Answer from the drawing. Dimensions are ordinates in mm from the lowest x, y and z of the part. A direction names the side the tool comes from. Give positions to 0.01 mm unless a question says otherwise; leave off trailing zeros. Write each loop counter-clockwise with the first axis right and the second up, starting at its lowest first coordinate (ties: lowest second). Pieces come first, ordered by that corner, then holes. Notation, with made-up numbers: (87.5, -9.5) -> (126.5, -9.5) arc R30 ccw to (126.5, 15.5) -> close; hole circle Ø2 at (10, 44). An arc over 180 degrees is marked (long way). Put each result on its own line as item: value. Start each with the question number.
1) A cutting plane is placed at A-A (z = 4.6). Write down the section's boundary in (x, y) (1 decimal), then the cut area to 3 significant figures.
2) Flat-ended cylindrical pins translate along their axes: pin 1 Ø1 at (x, z) = (11, 4) entering from -Y; pin 2 Ø3 at (x, y) = (5.5, 6.5) entering from +Z; pin 3 Ø1 at (x, y) = (9, 8.5) entering from +Z. Find the tip coordinate at first contact, or state that the pin passes through.
3) For the marked faces 1 and 2, determine the directions among +Z, -Z, +X, -X, +Y, -Y from which every point of the face is accessible in a straight line to the end or side of a thin tool.
4) A cutting plane is placed at C-C (x = 13.5). Write down the section's boundary in (y, z) (1 decimal), then the cut area to 3 significant figures.
5) A cutting plane is placed at D-D (x = 11.25). Write down the section's boundary in (y, z) (1 decimal).
6) Find the intervals of material crossed by line 1 along Y through (x, z) = (6.5, 4) (1 decimal); line 2 along X through (y, z) = (3.25, 3.3) (1 decimal); line 3 along X through (y, z) = (6.5, 0.7) (1 decimal), in increasing order. Write a range as from..to.
7) For a pull along X with two mould halves and no side action, classify the marked faces 3, 4, 5 and 6 as released by +X, released by -X, zero draft, split by the parting line, or undercut.
8) A cutting plane is placed at B-B (y = 8). Write down the section's boundary in (x, z) (1 decimal), then the cut area to 3 significant figures.
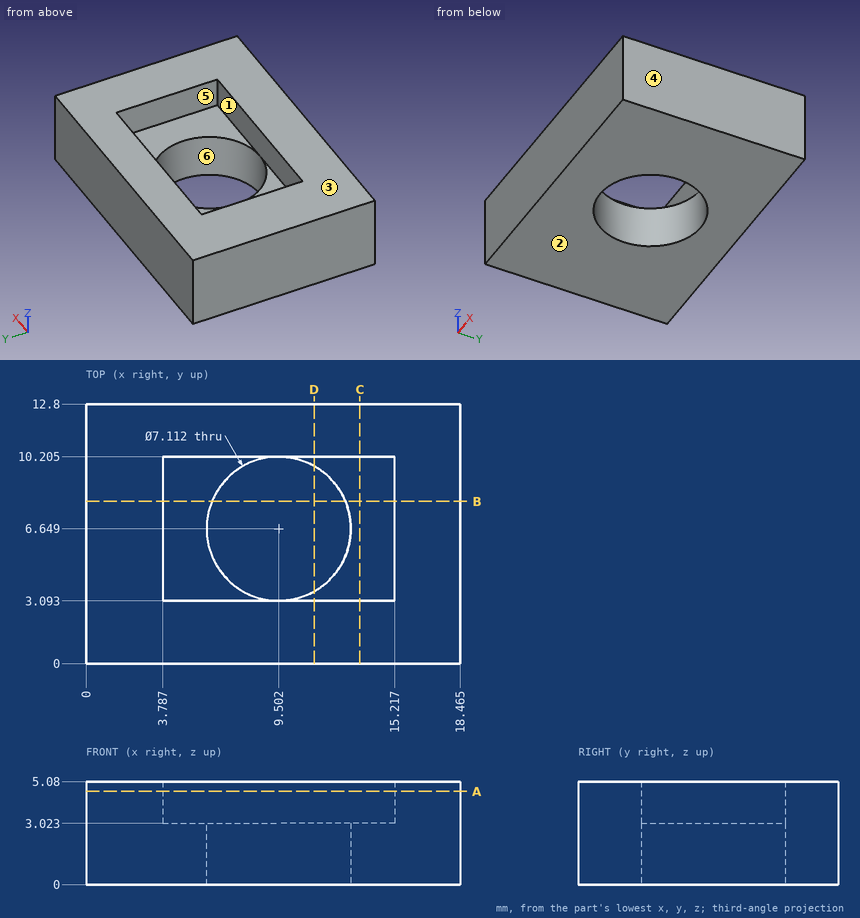
Reply:
1. outline: (0, 0) -> (18.5, 0) -> (18.5, 12.8) -> (0, 12.8) -> close; hole (3.8, 3.1) -> (15.2, 3.1) -> (15.2, 10.2) -> (3.8, 10.2) -> close
1. area: 155 mm2
2. pin 1: stops at y = 0
2. pin 2: stops at z = 3.02
2. pin 3: passes through
3. face 1: +Z
3. face 2: -Z, +X, -X, +Y, -Y
4. outline: (0, 0) -> (12.8, 0) -> (12.8, 5.1) -> (10.2, 5.1) -> (10.2, 3) -> (3.1, 3) -> (3.1, 5.1) -> (0, 5.1) -> close
4. area: 50.4 mm2
5. outline: (0, 0) -> (3.6, 0) -> (3.6, 3) -> (3.1, 3) -> (3.1, 5.1) -> (0, 5.1) -> close; (9.7, 0) -> (12.8, 0) -> (12.8, 5.1) -> (10.2, 5.1) -> (10.2, 3) -> (9.7, 3) -> close
6. line 1: y = 0..3.1, 10.2..12.8
6. line 2: x = 0..3.8, 15.2..18.5
6. line 3: x = 0..5.9, 13.1..18.5
7. face 3: zero draft
7. face 4: released by +X
7. face 5: undercut
7. face 6: undercut
8. outline: (0, 0) -> (6.2, 0) -> (6.2, 3) -> (3.8, 3) -> (3.8, 5.1) -> (0, 5.1) -> close; (12.8, 0) -> (18.5, 0) -> (18.5, 5.1) -> (15.2, 5.1) -> (15.2, 3) -> (12.8, 3) -> close
8. area: 50.4 mm2
